For this review, take the finished solid that the model builds, in its own axes (mm). Face numbers are marked on the shaded views. A direction names the side the tool comes from. Coordinates: 2 decimals unless noted, no trailing zeros. Write each loop counter-clockwise with the first axis right and the second up, starting at its lowest first coordinate (ties: lowest second). Pieces come first, ordered by that corner, then holes. Notation, with made-up numbers: M 49,86 L 101,86 A17 cw 101,97 Z; hole C 64.5,24 d10. An arc over 180 degrees is marked long. One line per question, with ' | ' between items.
from build123d import *

# Parameters (mm, degrees)
SKETCH1_W               = 16
SKETCH1_H               = 16
CCD_BASE_DEPTH          = 10
CCD_BASE_MOUNT_DEPTH    = 6
SKETCH5_R               = 6.35
LENSE_TUBE_DEPTH        = 10.16
SKETCH6_R               = 8.509
SKETCH6_R_2             = 5.842
LENSE_RIM_DEPTH         = 4.572
LENSE_GLASS_FACE_RADIUS = 5.842
LENSE_GLASS_HEIGHT      = 3.81


with BuildPart() as part:
    # Sketch1 → ccd_base (new body)
    with BuildSketch(Plane.XZ.offset(-1.6)):
        Rectangle(SKETCH1_W, SKETCH1_H)
    extrude(amount=-CCD_BASE_DEPTH)

    # Sketch2 → ccd_base_mount (add)
    with BuildSketch(Plane.XZ.offset(-1.6)):
        with BuildLine():
            Line((1.9, 9.75), (1.75, 9.75))
            ThreePointArc((1.75, 9.75), (0, 11.5), (-1.75, 9.75))
            Line((-1.75, 9.75), (-1.9, 9.75))
            Line((-1.9, 9.75), (-1.9, 8))
            Line((-1.9, 8), (1.9, 8))
            Line((1.9, 8), (1.9, 9.75))
        make_face()
    ccd_base_mount = extrude(amount=-CCD_BASE_MOUNT_DEPTH)

    # Mirror1: ccd_base_mount across plane
    add(ccd_base_mount.mirror(Plane.XY))

    # Sketch5 → lense_tube (add)
    with BuildSketch(Plane(origin=(0, 11.6, 0), x_dir=(1, 0, 0), z_dir=(0, 1, 0))):
        with Locations(Location((0, 0, 0), (0, 0, 90))):
            Circle(SKETCH5_R)
    extrude(amount=LENSE_TUBE_DEPTH)

    # Sketch6 → lense_rim (add)
    with BuildSketch(Plane(origin=(0, 21.76, 0), x_dir=(1, 0, 0), z_dir=(0, 1, 0))):
        with Locations(Location((0, 0, 0), (0, 0, 270))):
            Circle(SKETCH6_R)
        with Locations(Location((0, 0, 0), (0, 0, 270))):
            Circle(SKETCH6_R_2, mode=Mode.SUBTRACT)
    extrude(amount=LENSE_RIM_DEPTH)

    # lense_glass: an elliptical dome of height H over a round flat face of radius A is half a spheroid: the quarter ellipse of half axes A and H revolved about the face's axis
    with BuildSketch(Plane((0, 21.76, 0), x_dir=(0, 0, -1), z_dir=(1, 0, 0)), mode=Mode.PRIVATE) as lense_glass_quarter:
        Ellipse(LENSE_GLASS_FACE_RADIUS, LENSE_GLASS_HEIGHT)
        Rectangle(LENSE_GLASS_FACE_RADIUS, LENSE_GLASS_HEIGHT, align=(Align.MIN, Align.MIN), mode=Mode.INTERSECT)
    revolve(lense_glass_quarter.sketch, axis=Axis((0, 21.76, 0), (0, 1, 0)))


solid = part.part
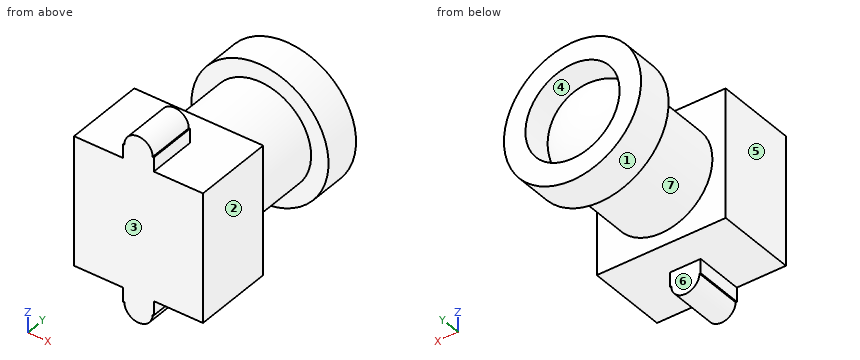
1. For line 1 along Y through (x, z) = (3, 7); line 2 along X through (y, z) = (22.9, 0); line 3 along X through (y, z) = (22.95, 0), list the stretches that pass through material, from the lowest coordinate up.
Computed values:
line 1: y = 1.6 to 11.6, 21.76 to 26.33 | line 2: x = -8.51 to -5.84, -5.57 to 5.57, 5.84 to 8.51 | line 3: x = -8.51 to -5.84, -5.55 to 5.55, 5.84 to 8.51
2. Draft analysis for pull direction X (two halves, no side actions). For the marked faces 1, 2, 3 and 4, state which applies: pulls with the +X half, pulls with the -X half, needs draft (parallel to the pull), parting line crosses it, or undercut.
Computed values:
face 1: parting line crosses it | face 2: pulls with the +X half | face 3: needs draft | face 4: undercut
3. Machinability: for the marked faces 5, 6 and 7, which of the approach directions +Z, -Z, +X, -X, +Y, -Y give a long, thin tool a straight path to every point of the face, cutting with its end or side? Answer none if there is none.
Computed values:
face 5: +Z, -Z, -X, -Y | face 6: -Z, +X, -X | face 7: none
4. Take a section at A-A on z = 7. State the section outline as (x, y) points, plus the area to 3 significant figures.
Computed values:
outline: M -8,1.6 L 8,1.6 L 8,11.6 L -8,11.6 Z; M -4.84,21.76 L 4.84,21.76 L 4.84,26.33 L -4.84,26.33 Z | area: 204 mm2
5. Clearance check with flat-ended pins moving along their axes: P1, Ø1, axis at x = 0, z = 10, coming from the +Y side; P2, Ø1.5, axis at y = 17.5, z = 0, coming from the +X side; P3, Ø3, axis at x = 5.5, y = 10.5, coming from the +Z side. State where each tip first meets the part, or that it passes through.
Computed values:
P1: stops at y = 7.6 | P2: stops at x = 6.35 | P3: stops at z = 8
6. Take a section at D-D on y = 13.75. State the section outline as (x, z) points, plus the area to 3 significant figures.
Computed values:
outline: C 0,0 d12.7 | area: 127 mm2
7. Take a section at B-B on y = 3.5. State the section outline as (x, z) points, plus the area to 3 significant figures.
Computed values:
outline: M -8,-8 L -1.9,-8 L -1.9,-9.75 L -1.75,-9.75 A1.75 ccw 1.75,-9.75 L 1.9,-9.75 L 1.9,-8 L 8,-8 L 8,8 L 1.9,8 L 1.9,9.75 L 1.75,9.75 A1.75 ccw -1.75,9.75 L -1.9,9.75 L -1.9,8 L -8,8 Z | area: 279 mm2
8. Take a section at C-C on x = -7. State the section outline as (y, z) points.
Computed values:
outline: M 1.6,-8 L 11.6,-8 L 11.6,8 L 1.6,8 Z; M 21.76,-4.84 L 26.33,-4.84 L 26.33,4.84 L 21.76,4.84 Z
